```python
from build123d import *

# Parameters (mm, degrees)
F0_W     = 150
F0_H     = 140
F1_DEPTH = 86
F3_DEPTH = 3
F2_R     = 2.5
F4_DEPTH = 6
F5_T     = -1.5
F6_W     = 19
F6_H     = 26
F7_DEPTH = 10
F8_R     = 10
F9_DEPTH = 5
F10_R    = 2


# Not quite as in the source:
# - a shell that OpenCascade refuses in one call is made with other operations: the cavity is built on its own and cut out


with BuildPart() as f1:
    # F0 (on Top) → F1 (new body)
    with BuildSketch(Plane.XY):
        Rectangle(F0_W, F0_H)
    extrude(amount=F1_DEPTH)

    # F2 (on face) → F3 (cut)
    with BuildSketch(Plane.XY.offset(86)):
        with BuildLine():
            Line((24.8082830088, 59), (-42.8082830088, 59))
            ThreePointArc((-42.8082830088, 59), (-57.0832611207, 48.0832611207), (-68, 33.8082830088))
            Line((-68, 33.8082830088), (-68, -33.8082830088))
            ThreePointArc((-68, -33.8082830088), (-57.0832611207, -48.0832611207), (-42.8082830088, -59))
            Line((-42.8082830088, -59), (24.8082830088, -59))
            ThreePointArc((24.8082830088, -59), (39.0832611207, -48.0832611207), (50, -33.8082830088))
            Line((50, -33.8082830088), (50, 33.8082830088))
            ThreePointArc((50, 33.8082830088), (39.0832611207, 48.0832611207), (24.8082830088, 59))
        make_face()
    extrude(amount=-F3_DEPTH, mode=Mode.SUBTRACT)

    # F2 (on face) → F4 (cut)
    with BuildSketch(Plane.XY.offset(86)):
        with Locations((-62, 53)):
            Circle(F2_R)
        with Locations((44, 53)):
            Circle(F2_R)
        with Locations((44, -53)):
            Circle(F2_R)
        with Locations((-62, -53)):
            Circle(F2_R)
    extrude(amount=-F4_DEPTH, mode=Mode.SUBTRACT)

    # F5: a shell. OpenCascade refuses it in one call, so the cavity is built on its own and cut out:
    # the body offset inwards by the wall thickness, plus a prism from it out through each open face.
    f5_core = offset(f1.part, amount=F5_T, kind=Kind.INTERSECTION, mode=Mode.PRIVATE)
    f5_exits = [f5_core.faces().sort_by_distance(p)[0] for p in [
        (-9, 0, 81.5),
    ]]
    add(f5_core, mode=Mode.SUBTRACT)
    extrude(f5_exits, amount=-F5_T, mode=Mode.SUBTRACT)

    # F6 (on face) → F7 (cut)
    with BuildSketch(Plane.XZ.offset(70)):
        with Locations((55.5, 49)):
            Rectangle(F6_W, F6_H)
    extrude(amount=-F7_DEPTH, mode=Mode.SUBTRACT)

    # F8 (on face) → F9 (cut)
    with BuildSketch(Plane(origin=(0, 70, 0), x_dir=(-1, 0, 0), z_dir=(0, 1, 0))):
        with Locations((-64, 56)):
            Circle(F8_R)
    extrude(amount=-F9_DEPTH, mode=Mode.SUBTRACT)

    # F10
    f10_edges = [f1.edges().sort_by_distance(p)[0] for p in [
        (75, 0, 86),
        (75, 0, 0),
        (-75, 0, 86),
        (-75, 0, 0),
    ]]
    fillet(f10_edges, radius=F10_R)


solid = f1.part
```
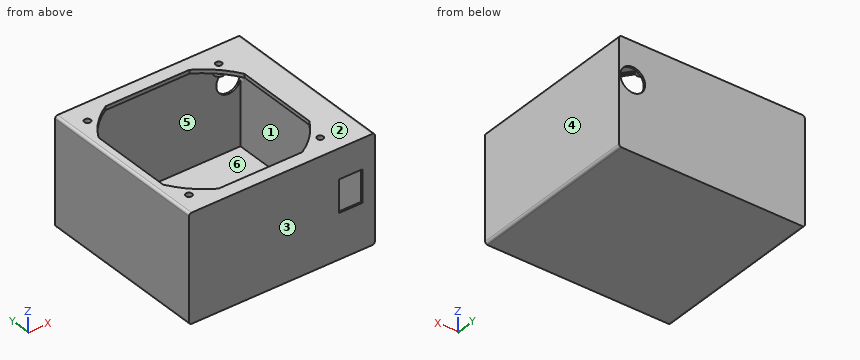
Can you work these out from the model? Positions are in its coordinate system, mm. Face numbers are marked on the shaded views. A direction names the side the tool comes from. Coordinates: 2 decimals unless noted, no trailing zeros. Write each loop counter-clockwise with the first axis right and the second up, starting at its lowest first coordinate (ties: lowest second). Pieces come first, ordered by that corner, then holes. Notation, with made-up numbers: M -13,57.5 L 38,57.5 A26 ccw 38,78.5 Z; hole C 38,-35 d2. An arc over 180 degrees is marked long. Answer as CSV lines item,"result".
Item 1: Imagine slicing it at C-C on y = -8.5. List the corners of the cut face in (x, z) for me, plus the area to 3 significant figures.
Geometry results:
outline,"M -75,2 A2 ccw -73,0 L 73,0 A2 ccw 75,2 L 75,84 A2 ccw 73,86 L 50,86 L 50,83 L 51.5,83 L 51.5,84.5 L 73.5,84.5 L 73.5,1.5 L -73.5,1.5 L -73.5,84.5 L -69.5,84.5 L -69.5,83 L -68,83 L -68,86 L -73,86 A2 ccw -75,84 Z"
area,"523 mm2"
Item 2: We'd pull the mould along X, two halves only. Please class the marked faces 3, 4, 5 and 6: +X half, -X half, draft (parallel to the pull), parting line (faces both ways), or undercut.
Geometry results:
face 3,"draft"
face 4,"+X half"
face 5,"undercut"
face 6,"undercut"
Item 3: On a 3-axis mill with a long thin cutter (end or side, diameter ignored), from which of +Z, -Z, +X, -X, +Y, -Y can I reach the whole of each face in a straight line? I mean the marked faces 1 and 2. Say none if no direction works.
Geometry results:
face 1,"none"
face 2,"+Z, +X, -X, +Y, -Y"
Item 4: Imagine slicing it at A-A on z = 56. List the corners of the cut face in (x, y) for me, plus the area to 3 significant figures.
Geometry results:
outline,"M -75,-70 L 46,-70 L 46,-68.5 L -73.5,-68.5 L -73.5,68.5 L 54,68.5 L 54,70 L -75,70 Z; M 65,-70 L 75,-70 L 75,70 L 74,70 L 74,65 L 73.5,65 L 73.5,-68.5 L 65,-68.5 Z"
area,"801 mm2"
Item 5: Please list where these lines run through material, in increasing order: line 1 along Y through (x, z) = (-62, 82); line 2 along X through (y, z) = (-33.5, 69); line 3 along Z through (x, y) = (54.5, 49).
Geometry results:
line 1,"y = -70 to -68.5, -57 to -55.5, -50.5 to -49, 49 to 50.5, 55.5 to 57, 68.5 to 70"
line 2,"x = -75 to -73.5, 73.5 to 75"
line 3,"z = 0 to 1.5, 84.5 to 86"
Item 6: I'm going to push flat-ended pins straight in: P1, Ø3, axis at x = -14.5, y = -20.5, coming from the +Z side; P2, Ø1.5, axis at x = -63, y = -52.5, coming from the +Z side. Where does each tip first touch, or does it pass through?
Geometry results:
P1,"stops at z = 1.5"
P2,"stops at z = 80"
Item 7: Imagine slicing it at B-B on z = 27. List the corners of the cut face in (x, y) for me, plus the area to 3 significant figures.
Geometry results:
outline,"M -75,-70 L 75,-70 L 75,70 L -75,70 Z; hole M -73.5,-68.5 L 73.5,-68.5 L 73.5,68.5 L -73.5,68.5 Z"
area,"861 mm2"
